```python
from build123d import *

# Parameters (mm, degrees)
SKETCH1_W           = 7
SKETCH1_H           = 2
BOSS_EXTRUDE1_DEPTH = 7
CUT_EXTRUDE1_DEPTH  = 3
SKETCH3_W           = 4
SKETCH3_H           = 1
CUT_EXTRUDE2_DEPTH  = 8
SKETCH4_W           = 3
SKETCH4_H           = 2
BOSS_EXTRUDE2_DEPTH = 3
BOSS_EXTRUDE4_DEPTH = 2
SKETCH7_R           = 2
CUT_EXTRUDE4_DEPTH  = 5


with BuildPart() as part:
    # Sketch1 → Boss-Extrude1 (new body)
    with BuildSketch(Plane.XY):
        Rectangle(SKETCH1_W, SKETCH1_H)
    extrude(amount=BOSS_EXTRUDE1_DEPTH)

    # Sketch2 → Cut-Extrude1 (cut, through all)
    with BuildSketch(Plane(origin=(0, 1, 0), x_dir=(1, 0, 0), z_dir=(0, 1, 0))):
        Polygon((3.5, -4), (-1.5, -7), (3.5, -7), align=None)
    extrude(amount=-CUT_EXTRUDE1_DEPTH, mode=Mode.SUBTRACT)

    # Sketch3 → Cut-Extrude2 (cut, through all)
    with BuildSketch(Plane.XY.offset(7)):
        with Locations((-0.5, -0.5)):
            Rectangle(SKETCH3_W, SKETCH3_H)
    extrude(amount=-CUT_EXTRUDE2_DEPTH, mode=Mode.SUBTRACT)

    # Sketch4 → Boss-Extrude2 (add)
    with BuildSketch(Plane(origin=(0, 1, 0), x_dir=(1, 0, 0), z_dir=(0, 1, 0))):
        with Locations((-2, -4)):
            Rectangle(SKETCH4_W, SKETCH4_H)
    extrude(amount=BOSS_EXTRUDE2_DEPTH)

    # Sketch6 → Boss-Extrude4 (add)
    with BuildSketch(Plane(origin=(0, 0, 3), x_dir=(-1, 0, 0), z_dir=(0, 0, -1))):
        with BuildLine():
            Line((0.5, 2), (0.5, 1))
            ThreePointArc((0.5, 1), (2.621320344, 1.878679656), (3.5, 4))
            Line((3.5, 4), (2.5, 4))
            ThreePointArc((2.5, 4), (1.914213562, 2.585786438), (0.5, 2))
        make_face()
        with BuildLine():
            Line((-2.5, 1), (0.5, 1))
            Line((0.5, 1), (0.5, 2))
            ThreePointArc((0.5, 2), (-0.914213562, 2.585786438), (-1.5, 4))
            Line((-1.5, 4), (-2.5, 4))
            Line((-2.5, 4), (-2.5, 1))
        make_face()
        with BuildLine():
            Line((2.5, 4), (3.5, 4))
            ThreePointArc((3.5, 4), (2.621320344, 6.121320344), (0.5, 7))
            Line((0.5, 7), (0.5, 6))
            ThreePointArc((0.5, 6), (1.914213562, 5.414213562), (2.5, 4))
        make_face()
        with BuildLine():
            ThreePointArc((3.5, 4), (2.621320344, 1.878679656), (0.5, 1))
            Line((0.5, 1), (3.5, 1))
            Line((3.5, 1), (3.5, 4))
        make_face()
    extrude(amount=BOSS_EXTRUDE4_DEPTH)

    # Sketch7 → Cut-Extrude4 (cut)
    with BuildSketch(Plane(origin=(0, 0, 1), x_dir=(-1, 0, 0), z_dir=(0, 0, -1))):
        with Locations((0.5, 4)):
            Circle(SKETCH7_R)
    extrude(amount=-CUT_EXTRUDE4_DEPTH, mode=Mode.SUBTRACT)


solid = part.part
```
For this review, take the finished solid that the model builds, in its own axes (mm). A direction names the side the tool comes from. Round coordinates to 2 decimals unless told otherwise and drop trailing zeros. Write each loop counter-clockwise with the first axis right and the second up, starting at its lowest first coordinate (ties: lowest second). Pieces come first, ordered by that corner, then holes. Notation, with made-up numbers: (46.25, 18.5) -> (94.25, 18.5) arc R19 cw to (94.25, 48.5) -> close; hole circle Ø11 at (45.25, 2). An arc over 180 degrees is marked (long way). Use one line per item in the form item = value.
Q1. The part is to be moulded in two halves that separate along X. For faces 1 (the flat face through (1.5, -0.5, 2.6)), 2 (the flat face through (2, 4, 2)), 3 (the flat face through (3.5, 0, 2)), say which applies: released by +X, released by -X, zero draft, split by the parting line, or undercut.
Resolved:
face_1 = undercut
face_2 = zero draft
face_3 = released by +X
Q2. Consider section B-B (x = 2.25). State the section outline as (y, z) points, then the cut area to 3 significant figures.
Resolved:
outline = (-1, 0) -> (1, 0) -> (1, 1) -> (4, 1) -> (4, 3) -> (1, 3) -> (1, 4.75) -> (-1, 4.75) -> close
area = 15.5 mm²
Q3. To check wall thickness, follow probe 1 along Y at (x, z) = (-3, 4.25); probe 2 along Y at (x, z) = (0.75, 4); probe 3 along Z at (x, y) = (-2.5, 5.75). State the ranges of each line that lie inside material, in increasing order. Write a range as from..to.
Resolved:
probe_1 = -1..4
probe_2 = 0..1
probe_3 = 1..3
Q4. Clearance check with flat-ended pins moving along their axes: pin 1 Ø0.5 at (y, z) = (1.5, 3.5) entering from +X; pin 2 Ø0.9 at (x, y) = (-1.5, 3) entering from +Z; pin 3 Ø0.8 at (x, z) = (-3, 4.5) entering from +Y; pin 4 Ø2 at (y, z) = (2.5, 2) entering from +X. State where each tip first meets the part, or that it passes through.
Resolved:
pin_1 = -0.5
pin_2 = through
pin_3 = 4
pin_4 = 2.5
Q5. Consider section D-D (z = 6.25). State the section outline as (x, y) points.
Resolved:
outline = (-3.5, -1) -> (-2.5, -1) -> (-2.5, 0) -> (-0.25, 0) -> (-0.25, 1) -> (-3.5, 1) -> close
Q6. Machinability: for faces 4 (the flat face through (-2, 2, 1)), 5 (the flat face through (-2, 2, 5)), 6 (the flat face through (2.5, 3, 2)), which of the approach directions +Z, -Z, +X, -X, +Y, -Y give a long, thin tool a straight path to every point of the face, cutting with its end or side? Answer none if there is none.
Resolved:
face_4 = -Z, +X, -X, +Y
face_5 = +Z, +X, -X, +Y
face_6 = +Z, -Z, +X, +Y
Q7. Consider section C-C (y = 1.75). State the section outline as (x, z) points.
Resolved:
outline = (-3.5, 1) -> (2.5, 1) -> (2.5, 3) -> (-0.5, 3) -> (-0.5, 5) -> (-3.5, 5) -> close
Q8. Consider section A-A (z = 0.5). State the section outline as (x, y) points.
Resolved:
outline = (-3.5, -1) -> (-2.5, -1) -> (-2.5, 0) -> (1.5, 0) -> (1.5, -1) -> (3.5, -1) -> (3.5, 1) -> (-3.5, 1) -> close
